Input: part model. Units: mm. Frame: model coordinates. Round coordinates to 2 decimals unless told otherwise and drop trailing zeros. Loops run counter-clockwise (first coordinate to the right, second up) from the corner with the lowest first, then second, coordinate; pieces in that order, holes last. Notation, with made-up numbers: (-26, 11) -> (-13, 11) arc R17 cw to (-13, 37) -> close; hole circle Ø7 at (26.5, 24). An arc over 180 degrees is marked (long way). One line per question, with ' | ' between items. Start each with the question number.
Q1. Material intervals for L1, parallel to Y at x = -30, z = 3.1; L2, parallel to X at y = 243, z = 0.4; L3, parallel to Y at x = -93, z = 3.55, sorted ascending.
Q2. Contact query for flat-ended pins moving along their axis: P1, Ø12, axis at x = -33, y = 235.5, coming from the +Z side; P2, Ø10, axis at x = -58, y = 120.5, coming from the -Z side. Output: stop coordinate, or through.
Q3. Cut plane B-B on x = -32.5. Return loops of the section in (y, z).
Q4. Cut plane C-C on z = 4.05. Return loops of the section in (x, y).
Q5. Cut plane A-A on y = 249. Return loops of the section in (x, z), and give its area (3 significant figures).
from build123d import *

# Parameters (mm, degrees)
SKETCH1_W           = 112
SKETCH1_H           = 280
SKETCH1_W_2         = 82
SKETCH1_H_2         = 40
BOSS_EXTRUDE1_DEPTH = 5
FILLET1_R           = 20
FILLET2_R           = 10


with BuildPart() as part:
    # Sketch1 → Boss-Extrude1 (new body)
    with BuildSketch(Plane.XY):
        with Locations((-56, 140)):
            Rectangle(SKETCH1_W, SKETCH1_H)
        with Locations((-56, 245)):
            Rectangle(SKETCH1_W_2, SKETCH1_H_2, mode=Mode.SUBTRACT)
    extrude(amount=BOSS_EXTRUDE1_DEPTH)

    # Fillet1
    fillet1_edges = [part.edges().sort_by_distance(p)[0] for p in [
        (-112, 280, 2.5),
        (0, 280, 2.5),
    ]]
    fillet(fillet1_edges, radius=FILLET1_R)

    # Fillet2
    fillet2_edges = [part.edges().sort_by_distance(p)[0] for p in [
        (-15, 225, 2.5),
        (-15, 265, 2.5),
        (-97, 265, 2.5),
        (-97, 225, 2.5),
    ]]
    fillet(fillet2_edges, radius=FILLET2_R)


solid = part.part
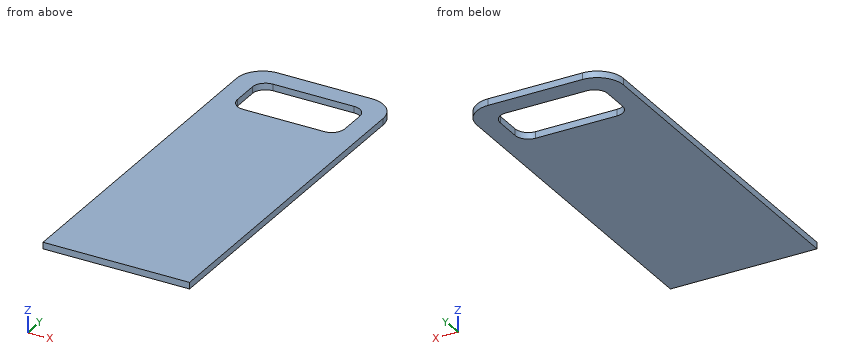
Results:
1) L1: 0 to 225, 265 to 280 | L2: -112 to -97, -15 to 0 | L3: 0 to 227, 263 to 279.97
2) P1: through | P2: z = 0
3) outline: (0, 0) -> (225, 0) -> (225, 5) -> (0, 5) -> close; (265, 0) -> (280, 0) -> (280, 5) -> (265, 5) -> close
4) outline: (-112, 0) -> (0, 0) -> (0, 260) arc R20 ccw to (-20, 280) -> (-92, 280) arc R20 ccw to (-112, 260) -> close; hole (-97, 235) arc R10 ccw to (-87, 225) -> (-25, 225) arc R10 ccw to (-15, 235) -> (-15, 255) arc R10 ccw to (-25, 265) -> (-87, 265) arc R10 ccw to (-97, 255) -> close
5) outline: (-112, 0) -> (-97, 0) -> (-97, 5) -> (-112, 5) -> close; (-15, 0) -> (0, 0) -> (0, 5) -> (-15, 5) -> close | area: 150 mm^2
